```python
from build123d import *

# Parameters (mm, degrees)
F0_R     = 10.5
F0_R_2   = 9.25
F1_DEPTH = 10
F3_DEPTH = 12.5


with BuildPart() as f1:
    # F0 (on Top) → F1 (new body)
    with BuildSketch(Plane.XY):
        Circle(F0_R)
        Circle(F0_R_2, mode=Mode.SUBTRACT)
    extrude(amount=F1_DEPTH)

    # F2 (on Front) → F3 (cut, symmetric)
    with BuildSketch(Plane.XZ):
        with BuildLine():
            add(Edge.make_bspline(
                [(11.2434588373, 10.0891618058), (11.0047016615, 10.1132977758), (10.7632299901, 10.112965479), (10.5204237755, 10.0891618058)],
                knots=[0, 0, 0, 0, 0.0562635786, 0.0562635786, 0.0562635786, 0.0562635786], degree=3))
            Line((10.5204237755, 10.0891618058), (11.2434588373, 10.0891618058))
        make_face()
        with BuildLine():
            Line((10.5204237755, 10.0891618058), (-10.5204237755, 10.0891618058))
            add(Edge.make_bspline(
                [(-10.5204237755, 10.0891618058), (-9.8416288611, 10.0226156826), (-8.0921208581, 9.3880562532), (-5.7194913073, 6.93683362), (-4.2906021774, 5.397823396), (-1.4143970077, 5.0322200394), (-0.6250849692, 5.0027752295), (0, 5)],
                knots=[0.0562635786, 0.0562635786, 0.0562635786, 0.0562635786, 0.2135553971, 0.4555283654, 0.6401415553, 0.844289529, 1, 1, 1, 1], degree=3))
            add(Edge.make_bspline(
                [(10.5204237755, 10.0891618058), (9.8416288611, 10.0226156826), (8.0921208581, 9.3880562532), (5.7194913073, 6.93683362), (4.2906021774, 5.397823396), (1.4143970077, 5.0322200394), (0.6250849692, 5.0027752295), (0, 5)],
                knots=[0.0562635786, 0.0562635786, 0.0562635786, 0.0562635786, 0.2135553971, 0.4555283654, 0.6401415553, 0.844289529, 1, 1, 1, 1], degree=3))
        make_face()
        with BuildLine():
            add(Edge.make_bspline(
                [(-11.2434588373, 10.0891618058), (-11.0047016615, 10.1132977758), (-10.7632299901, 10.112965479), (-10.5204237755, 10.0891618058)],
                knots=[0, 0, 0, 0, 0.0562635786, 0.0562635786, 0.0562635786, 0.0562635786], degree=3))
            Line((-11.2434588373, 10.0891618058), (-10.5204237755, 10.0891618058))
        make_face()
    extrude(amount=F3_DEPTH, both=True, mode=Mode.SUBTRACT)


solid = f1.part
```
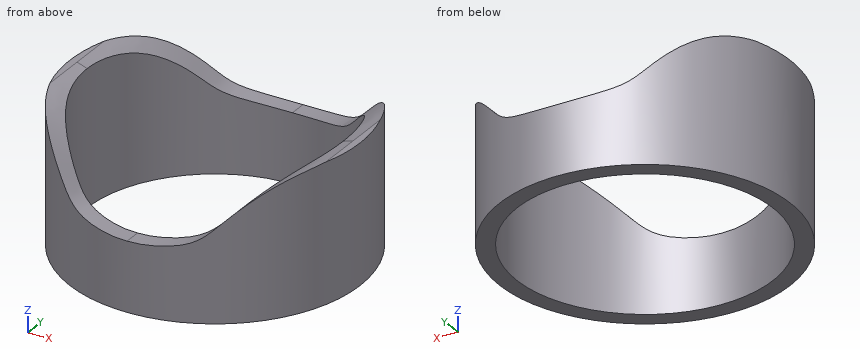
Verification items for the finished model (mm, model axes). Give positions to 0.01 mm unless a question says otherwise; leave off trailing zeros. Order: outer loops, then holes, each group sorted by start corner. A loop starts at its lowest first (then second) coordinate and runs counter-clockwise, first axis right, second up. Notation, with made-up numbers: M -19,-20.5 L -14,-20.5 A28 cw -14,-0.5 Z; hole C -28.75,73 d11. An arc over 180 degrees is marked long. Answer in a Markdown table with one row per item. Add a question column.
Item 1: Scan lines: probe 1 along X at (y, z) = (0, 4); probe 2 along X at (y, z) = (5.75, 9.25). Record each from-to range of solid material in increasing order. Write a range as from..to.
Item 2: Section check A-A, the plane z = 3.5. Enter the section's corners in (x, y), and give its area (3 significant figures).
Item 3: Gauge pin test, flat ends, axial feed: pin 1 (6 mm diameter, centred on y = 4, z = 8.5, fed in from +X); pin 2 (1.5 mm diameter, centred on y = 2.5, z = 6, fed in from +X); pin 3 (5 mm diameter, centred on y = -4.5, z = 6.5, fed in from +X); pin 4 (4 mm diameter, centred on x = -5.5, y = 6, fed in from -Z). Record the tip position at first contact, or that the pin passes through.
Filled sheet:
| question | item | result |
|---|---|---|
| 1 | probe 1 | x = -10.5..-9.25, 9.25..10.5 |
| 1 | probe 2 | x = -8.79..-8.31, 8.31..8.79 |
| 2 | outline | C 0,0 d21; hole C 0,0 d18.5 |
| 2 | area | 77.6 mm^2 |
| 3 | pin 1 | stops at x = 10.45 |
| 3 | pin 2 | stops at x = 10.35 |
| 3 | pin 3 | stops at x = 10.31 |
| 3 | pin 4 | stops at z = 0 |
